Source: CAD feature listing. Evaluate the final solid. Frame: model axes, mm. Face numbers are marked on the shaded views. A direction names the side the tool comes from. Give positions to 0.01 mm unless a question says otherwise; leave off trailing zeros. Answer as a JSON object with one key per item and string values. Group by question number.
Item 1: Ray query, probe 1 along Z at (x, y) = (-172, 64.5); probe 2 along Y at (x, z) = (-135, 185); probe 3 along Y at (x, z) = (-136, 185). Return the intervals inside material, ascending. Write a range as from..to.
Item 2: Pull-direction query (Y, two-part tool) for the marked faces 1, 2 and 3; classes: pulls with the +Y half, pulls with the -Y half, needs draft (parallel to the pull), parting line crosses it, or undercut.
Item 3: Access query for the marked faces 4, 5 and 6. Directions: +Z, -Z, +X, -X, +Y, -Y. A direction counts if a zero-diameter tool reaches every point of the face in a straight line with its end or side. Return the directions, or none.
Item 4: First-contact query: pin 1 Ø9 at (y, z) = (168.93, 185) entering from -X; pin 2 Ø5.5 at (x, z) = (-174, 141) entering from -Y; pin 3 Ø6 at (x, z) = (-125, 190) entering from +Y. Flat tips, straight axial feed; report the tip coordinate or a pass-through.
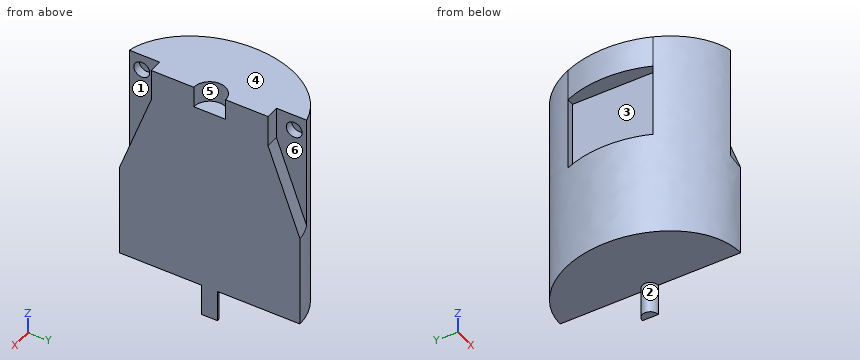
from build123d import *

# Parameters (mm, degrees)
CROQUIS1_RX             = 85
CROQUIS1_RY             = 67.73101263
SALIENTE_EXTRUIR1_DEPTH = 200
CORTAR_EXTRUIR1_DEPTH   = 100
SALIENTE_EXTRUIR2_DEPTH = 30
CROQUIS5_R              = 7.5
SALIENTE_EXTRUIR3_DEPTH = 30
CORTAR_EXTRUIR3_DEPTH   = 30
CROQUIS8_W              = 83.299216536
CROQUIS8_H              = 210.979163193
CORTAR_EXTRUIR4_DEPTH   = 348.816388214
CROQUIS9_R              = 15
CORTAR_EXTRUIR5_DEPTH   = 20
CROQUIS10_R             = 7.5
CORTAR_EXTRUIR6_DEPTH   = 8
CORTAR_EXTRUIR7_DEPTH   = 12.5


with BuildPart() as part:
    # Croquis1 → Saliente-Extruir1 (new body)
    with BuildSketch(Plane.XY):
        with Locations(Location((-119.067557665, 97.160736636), (0, 0, 90))):
            Ellipse(CROQUIS1_RX, CROQUIS1_RY)
    extrude(amount=SALIENTE_EXTRUIR1_DEPTH)

    # Croquis3 → Cortar-Extruir1 (cut)
    with BuildSketch(Plane.XY.offset(200)):
        with BuildLine():
            Line((-171.829854236, 137.159885706), (-171.829854236, 57.159885706))
            Line((-171.829854236, 57.159885706), (-178.829854236, 57.159885706))
            add(Edge.make_bspline(
                [(-178.830577491, 137.159885706), (-195.829371976, 97.159643663), (-178.829854236, 57.159885706)],
                knots=[1.080850346, 1.080850346, 1.080850346, 2.060764999, 2.060764999, 2.060764999], degree=2, weights=[1, 0.882352941, 1]))
            Line((-178.830577491, 137.159885706), (-171.829854236, 137.159885706))
        make_face()
    extrude(amount=-CORTAR_EXTRUIR1_DEPTH, mode=Mode.SUBTRACT)

    # Croquis4 → Saliente-Extruir2 (add)
    with BuildSketch(Plane.XY.offset(200)):
        with BuildLine():
            Line((-178.830577491, 137.159885706), (-171.829854236, 137.159885706))
            Line((-171.829854236, 137.159885706), (-171.829854236, 57.159885706))
            Line((-171.829854236, 57.159885706), (-178.829854236, 57.159885706))
            add(Edge.make_bspline(
                [(-178.830577491, 137.159885706), (-195.797797403, 97.186782087), (-178.829854236, 57.159885706)],
                knots=[4.219557052, 4.219557052, 4.219557052, 5.198274326, 5.198274326, 5.198274326], degree=2, weights=[1, 0.882634519, 1]))
        make_face()
    extrude(amount=-SALIENTE_EXTRUIR2_DEPTH)

    # Croquis5 → Saliente-Extruir3 (add)
    with BuildSketch(Plane(origin=(0, 0, 0), x_dir=(-1, 0, 0), z_dir=(0, 0, -1))):
        with Locations(Location((119.067557665, 97.160736636, 0), (0, 0, 180))):
            Circle(CROQUIS5_R)
    extrude(amount=SALIENTE_EXTRUIR3_DEPTH)

    # Croquis7 → Cortar-Extruir3 (cut)
    with BuildSketch(Plane.XY.offset(200)):
        with BuildLine():
            Line((-131.567557665, 42.160736636), (-106.567557665, 42.160736636))
            Line((-106.567557665, 42.160736636), (-106.567557665, 13.620827843))
            add(Edge.make_bspline(
                [(-131.567557665, 13.620827843), (-119.067557665, 10.675126293), (-106.567557665, 13.620827843)],
                knots=[6.0975677, 6.0975677, 6.0975677, 6.468802915, 6.468802915, 6.468802915], degree=2, weights=[1, 0.982822456, 1]))
            Line((-131.567557665, 13.620827843), (-131.567557665, 42.160736636))
        make_face()
        with BuildLine():
            Line((-131.567557665, 180.700645429), (-131.567557665, 152.160736636))
            Line((-131.567557665, 152.160736636), (-106.567557665, 152.160736636))
            Line((-106.567557665, 152.160736636), (-106.567557665, 180.700645429))
            add(Edge.make_bspline(
                [(-106.567557665, 180.700645429), (-119.067557665, 183.64634698), (-131.567557665, 180.700645429)],
                knots=[2.955975046, 2.955975046, 2.955975046, 3.327210261, 3.327210261, 3.327210261], degree=2, weights=[1, 0.982822456, 1]))
        make_face()
    extrude(amount=-CORTAR_EXTRUIR3_DEPTH, mode=Mode.SUBTRACT)

    # Croquis8 → Cortar-Extruir4 (cut, through all)
    with BuildSketch(Plane.XY.offset(200)):
        with Locations((-77.417949397, 96.990041521)):
            Rectangle(CROQUIS8_W, CROQUIS8_H)
    extrude(amount=-CORTAR_EXTRUIR4_DEPTH, mode=Mode.SUBTRACT)

    # Croquis9 → Cortar-Extruir5 (cut)
    with BuildSketch(Plane.XY.offset(200)):
        with Locations((-119.067557665, 97.160736636)):
            Circle(CROQUIS9_R)
    extrude(amount=-CORTAR_EXTRUIR5_DEPTH, mode=Mode.SUBTRACT)

    # Croquis10 → Cortar-Extruir6 (cut)
    with BuildSketch(Plane(origin=(-131.567557665, 0, 0), x_dir=(0, 0, -1), z_dir=(1, 0, 0))):
        with Locations((-185, 168.930691033)):
            Circle(CROQUIS10_R)
        with Locations((-185, 25.39078224)):
            Circle(CROQUIS10_R)
    extrude(amount=-CORTAR_EXTRUIR6_DEPTH, mode=Mode.SUBTRACT)

    # Croquis11 → Cortar-Extruir7 (cut)
    with BuildSketch(Plane(origin=(-119.067557665, 0, 0), x_dir=(0, 0, -1), z_dir=(1, 0, 0))):
        Polygon((-170, 42.160736636), (-57.236885506, 1.118319437), (-170, -2.441940529), align=None)
        Polygon((-170, 152.160736636), (-58.81920935, 192.627235055), (-170, 211.002181537), align=None)
    extrude(amount=-CORTAR_EXTRUIR7_DEPTH, mode=Mode.SUBTRACT)


solid = part.part
Worked answers:
{
 "1": {"probe 1": "0..100, 170..200", "probe 2": "14.55..17.89, 32.89..161.43, 176.43..179.78", "probe 3": "14.86..17.89, 32.89..161.43, 176.43..179.46"},
 "2": {"face 1": "needs draft", "face 2": "parting line crosses it", "face 3": "undercut"},
 "3": {"face 4": "+Z, +X, -X, +Y, -Y", "face 5": "+Z, +X", "face 6": "+Z, +X, +Y"},
 "4": {"pin 1": "x = -160.47", "pin 2": "y = 42.97", "pin 3": "y = 152.16"}
}
